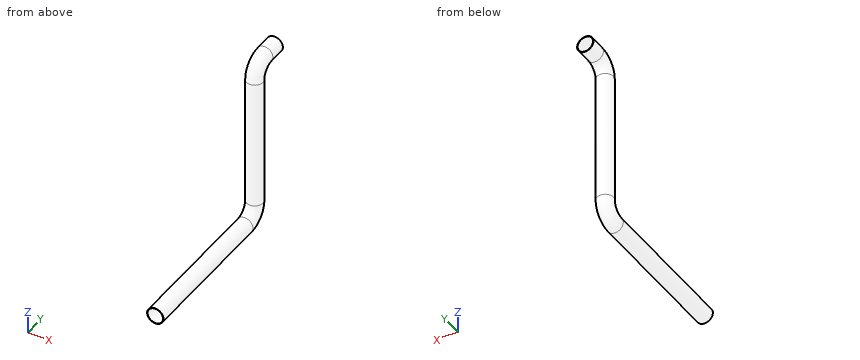
from build123d import *

# Parameters (mm, degrees)
F0_R   = 25
F0_R_2 = 23.5


with BuildPart() as f2:
    # F2: sweep along a path in F1
    with BuildLine(Plane.YZ) as f2_path:
        Line((0, 0), (-50, 0))
        ThreePointArc((-50, 0), (-85.355339, -14.644661), (-100, -50))
        Line((-100, -50), (-100, -450))
        ThreePointArc((-100, -450), (-114.644661, -485.355339), (-150, -500))
        Line((-150, -500), (-600, -500))
    # F0 (on Front) → F2 (sweep)
    with BuildSketch(Plane.XZ):
        Circle(F0_R)
        Circle(F0_R_2, mode=Mode.SUBTRACT)
    sweep(path=f2_path.line)


solid = f2.part
CAD build for the part. Positions are in the model's coordinates, mm. Round coordinates to 2 decimals unless told otherwise and drop trailing zeros. Write each loop counter-clockwise with the first axis right and the second up, starting at its lowest first coordinate (ties: lowest second). Pieces come first, ordered by that corner, then holes. Notation, with made-up numbers: M -21,64 L 9,64 A17 ccw 9,70 Z; hole C -31,46 d7. An arc over 180 degrees is marked long. Use a Markdown table: item, result. Add a question column.
1. Slice it at A-A on y = -395. Give the cut face in (x, z).
2. Flat gauge pins, fed straight in: P1, Ø12, axis at x = -13, y = -267, coming from the +Z side; P2, Ø6, axis at y = -111.5, z = -80, coming from the +X side; P3, Ø1.5, axis at x = -4.5, y = -197.5, coming from the -Z side. Where does each tip first touch, or does it go through?
3. Drill centre lines: probe 1 along Z at (x, y) = (0, -471); probe 2 along Z at (x, y) = (0, -38.5); probe 3 along X at (y, z) = (-108.5, -213). Where is each one in solid material? Low to high.
Reply:
| question | item | result |
|---|---|---|
| 1 | outline | C 0,-500 d50; hole C 0,-500 d47 |
| 2 | P1 | stops at z = -476 |
| 2 | P2 | stops at x = 23.51 |
| 2 | P3 | stops at z = -524.72 |
| 3 | probe 1 | z = -525 to -523.5, -476.5 to -475 |
| 3 | probe 2 | z = -25 to -23.5, 23.5 to 25 |
| 3 | probe 3 | x = -23.51 to -21.91, 21.91 to 23.51 |
